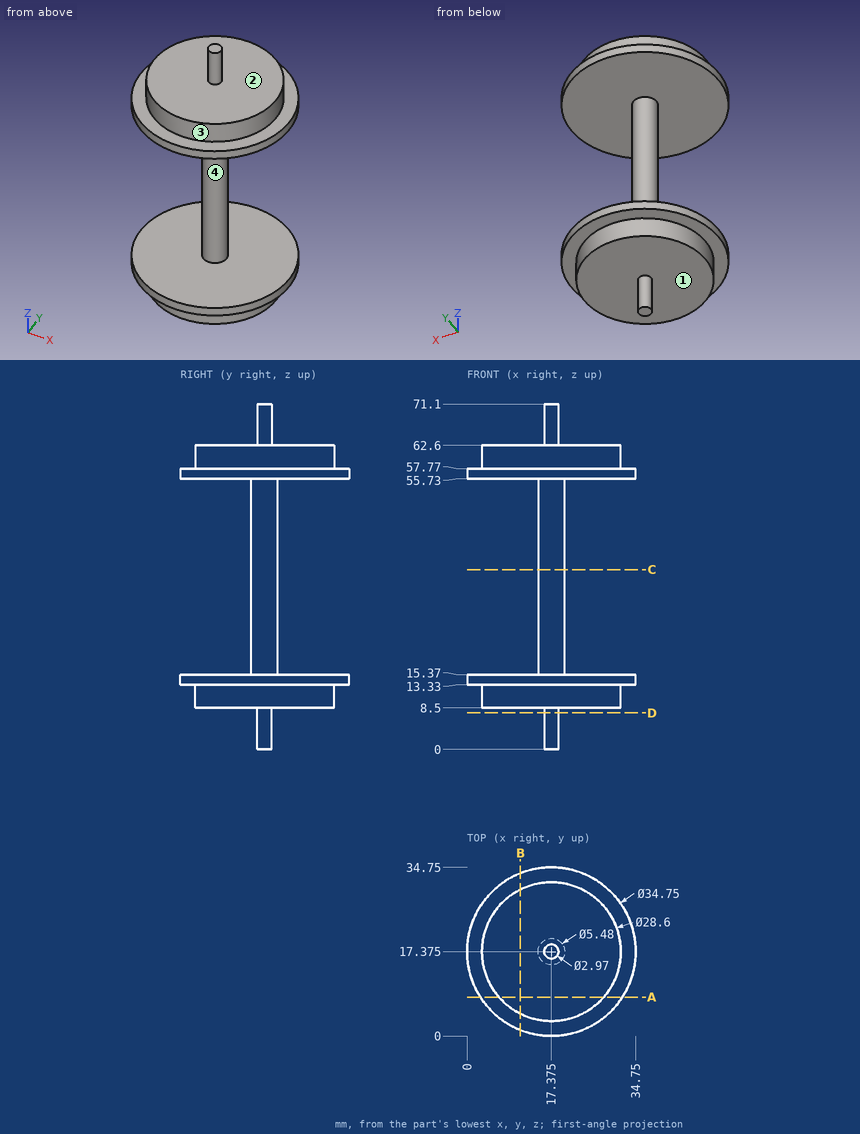
Here's the drawing with two shaded views (mm, measured from the low corner). I have some questions. Coordinates: 2 decimals unless noted, no trailing zeros. Order: outer loops, then holes, each group sorted by start corner. A loop starts at its lowest first (then second) coordinate and runs counter-clockwise, first axis right, second up.
Q1. Suppose I cut it at B-B on x = 11. Please give me the cut outline in (y, z), and give its area (3 significant figures).
Q2. Suppose I cut it at C-C on z = 37. Please give me the cut outline in (x, y) (3 decimals).
Q3. Suppose I cut it at A-A on y = 8. Please give me the cut outline in (x, z).
Q4. Suppose I cut it at D-D on z = 7.5. Please give me the cut outline in (x, y) (3 decimals), and give its area (3 significant figures).
Q5. Please list where these lines run through material, in increasing order: L1, parallel to Z at x = 24.5, y = 25.5; L2, parallel to Z at x = 16, y = 33; L3, parallel to X at y = 18, z = 40.
Q6. Thinking about a two-plate mould opening in Z: for the marked faces 1, 2, 3 and 4, which applies, released by +Z, released by -Z, zero draft, split by the parting line, or undercut?
Q7. Will these pins go through, and if not, where does the flat tip stop? pin 1 (5 mm diameter, centred on x = 24.5, y = 19, fed in from -Z); pin 2 (1 mm diameter, centred on x = 20, y = 12, fed in from +Z); pin 3 (8 mm diameter, centred on y = 11.5, z = 33.5, fed in from -X).
Answer:
1. outline: (1.21, 13.33) - (4.57, 13.33) - (4.57, 8.5) - (30.18, 8.5) - (30.18, 13.33) - (33.54, 13.33) - (33.54, 15.37) - (1.21, 15.37) - close; (1.21, 55.73) - (33.54, 55.73) - (33.54, 57.77) - (30.18, 57.77) - (30.18, 62.6) - (4.57, 62.6) - (4.57, 57.77) - (1.21, 57.77) - close
1. area: 379 mm2
2. outline: circle Ø5.48 at (17.375, 17.375)
3. outline: (2.75, 13.33) - (6.58, 13.33) - (6.58, 8.5) - (28.17, 8.5) - (28.17, 13.33) - (32, 13.33) - (32, 15.37) - (2.75, 15.37) - close; (2.75, 55.73) - (32, 55.73) - (32, 57.77) - (28.17, 57.77) - (28.17, 62.6) - (6.58, 62.6) - (6.58, 57.77) - (2.75, 57.77) - close
4. outline: circle Ø2.97 at (17.375, 17.375)
4. area: 6.93 mm2
5. L1: z = 8.5 to 15.37, 55.73 to 62.6
5. L2: z = 13.33 to 15.37, 55.73 to 57.77
5. L3: x = 14.71 to 20.04
6. face 1: released by -Z
6. face 2: released by +Z
6. face 3: zero draft
6. face 4: undercut
7. pin 1: stops at z = 8.5
7. pin 2: stops at z = 62.6
7. pin 3: stops at x = 15.38
